from build123d import *

# Parameters (mm, degrees)
SKETCH_1_R               = 17.25
EXTRUDE_1_DEPTH          = 14
SKETCH_2_R               = 31
EXTRUDE_2_DEPTH          = 10
CUT_EXTRUDE_1_DEPTH      = 50.979995998
CUT_EXTRUDE_1_DEPTH_BACK = 50.979995998
SKETCH_3_W               = 21
SKETCH_3_H               = 21
EXTRUDE_3_DEPTH          = 20
SKETCH_5_W               = 21
SKETCH_5_H               = 21
CUT_EXTRUDE_2_DEPTH      = 20
SKETCH_6_R               = 1.65
CUT_EXTRUDE_3_DEPTH      = 56
EXTRUDE_4_DEPTH          = 5


with BuildPart() as part:
    # 草图1 → 凸台-拉伸1 (new body)
    with BuildSketch(Plane.XY):
        Circle(SKETCH_1_R)
    extrude(amount=EXTRUDE_1_DEPTH)

    # 草图2 → 凸台-拉伸2 (add)
    with BuildSketch(Plane.XY.offset(14)):
        Circle(SKETCH_2_R)
    extrude(amount=EXTRUDE_2_DEPTH)

    # 草图3 → 切除-拉伸1 (cut, two sides: drawn at the far end of the back side and taken through both)
    with BuildSketch(Plane(origin=(0, 0, 0), x_dir=(-1, 0, 0), z_dir=(0, 0, -1)).offset(-CUT_EXTRUDE_1_DEPTH_BACK)):
        Rectangle(SKETCH_3_W, SKETCH_3_H)
    extrude(amount=CUT_EXTRUDE_1_DEPTH + CUT_EXTRUDE_1_DEPTH_BACK, mode=Mode.SUBTRACT)

    # 草图4 → 凸台-拉伸3 (add)
    with BuildSketch(Plane.XY.offset(24)):
        with BuildLine():
            Line((-12.959637187, 15.233115373), (13.493683466, 14.762130826))
            ThreePointArc((13.493683466, 14.762130826), (20, 0), (13.493683466, -14.762130826))
            Line((13.493683466, -14.762130826), (-12.959637187, -15.233115373))
            ThreePointArc((-12.959637187, -15.233115373), (-20, 0), (-12.959637187, 15.233115373))
        make_face()
    extrude(amount=EXTRUDE_3_DEPTH)

    # 草图5 → 切除-拉伸2 (cut)
    with BuildSketch(Plane(origin=(0, 0, 24), x_dir=(-1, 0, 0), z_dir=(0, 0, -1))):
        Rectangle(SKETCH_5_W, SKETCH_5_H)
    extrude(amount=-CUT_EXTRUDE_2_DEPTH, mode=Mode.SUBTRACT)

    # 草图6 → 切除-拉伸3 (cut)
    with BuildSketch(Plane(origin=(0.267023139, 14.9976231, 0), x_dir=(0.9998415399853875, -0.017801542619919335, 0), z_dir=(0.017801542619919338, 0.9998415399853876, 0))):
        with Locations((0, -34)):
            Circle(SKETCH_6_R)
    extrude(amount=-CUT_EXTRUDE_3_DEPTH, mode=Mode.SUBTRACT)

    # 草图8 → 凸台-拉伸4 (add)
    with BuildSketch(Plane.XY.offset(44)):
        with BuildLine():
            Line((-12.959637187, -15.233115373), (13.493683466, -14.762130826))
            ThreePointArc((13.493683466, -14.762130826), (20, 0), (13.493683466, 14.762130826))
            Line((13.493683466, 14.762130826), (-12.959637187, 15.233115373))
            ThreePointArc((-12.959637187, 15.233115373), (-20, 0), (-12.959637187, -15.233115373))
        make_face()
    extrude(amount=EXTRUDE_4_DEPTH)


solid = part.part
CAD build for the part. Positions are in the model's coordinates, mm. A direction names the side the tool comes from. Give positions to 0.01 mm unless a question says otherwise; leave off trailing zeros. Loops run counter-clockwise (first coordinate to the right, second up) from the corner with the lowest first, then second, coordinate; pieces in that order, holes last. Notation, with made-up numbers: M 71,86 L 85,86 A18 cw 85,99 Z; hole C -2,13 d7. An arc over 180 degrees is marked long. Answer in a Markdown table with one row per item. Add a question column.
Item 1: Band-saw the part on C-C on z = 13. Give the cut face in (x, y), then the cut area to 3 significant figures.
Item 2: Band-saw the part on A-A on z = 39. Give the cut face in (x, y), then the cut area to 3 significant figures.
Item 3: Tool access for faces 5 (the face through (20, 0, 36)), 6 (the face through (-4.036, 30.736, 18.93)), 7 (the face through (10.5, 0, 22)): list every direction of +Z, -Z, +X, -X, +Y, -Y with a clear straight run to the whole face (end or side of a thin tool).
Item 4: Probe probe 1 along X at (y, z) = (-0.5, 9); probe 2 along X at (y, z) = (4, 2); probe 3 along Y at (x, z) = (0, 42.5). List the from-to ranges inside material, lowest first.
Item 5: Band-saw the part on B-B on y = 0. Give the cut face in (x, z).
Item 6: Mould opens along Y. For faces 1 (the face through (0, -20, 24)), 2 (the face through (0, -10.5, 22)), 3 (the face through (0, 10.5, 22)), 4 (the face through (-20, 0, 36)) say: +Y half, -Y half, draft (parallel to the pull), parting line (faces both ways), or undercut.
Item 7: Band-saw the part on D-D on x = 0. Give the number of separate pieces and of enclosed holes in the cut face, then the cut area to 3 significant figures.
Item 8: Drop flat-ended pins along their axis: P1, Ø1, axis at x = 6.5, z = 6, coming from the +Y side; P2, Ø4, axis at y = 11.5, z = 44, coming from the -X side; P3, Ø10, axis at x = 19.5, y = -12, coming from the -Z side. Give the stop position or say it passes through.
Reply:
| question | item | result |
|---|---|---|
| 1 | outline | C 0,0 d34.5; hole M -10.5,-10.5 L 10.5,-10.5 L 10.5,10.5 L -10.5,10.5 Z |
| 1 | area | 494 mm^2 |
| 2 | outline | M -12.96,-15.23 L 13.49,-14.76 A20 ccw 13.49,14.76 L -12.96,15.23 A20 ccw Z; hole M -10.5,-10.5 L 10.5,-10.5 L 10.5,10.5 L -10.5,10.5 Z |
| 2 | area | 634 mm^2 |
| 3 | face 5 | +Z, +X |
| 3 | face 6 | +Z, -Z |
| 3 | face 7 | -Z |
| 4 | probe 1 | x = -17.24 to -10.5, 10.5 to 17.24 |
| 4 | probe 2 | x = -16.78 to -10.5, 10.5 to 16.78 |
| 4 | probe 3 | y = -15 to -10.5, 10.5 to 15 |
| 5 | outline | M -31,14 L -17.25,14 L -17.25,0 L -10.5,0 L -10.5,44 L 10.5,44 L 10.5,0 L 17.25,0 L 17.25,14 L 31,14 L 31,24 L 20,24 L 20,49 L -20,49 L -20,24 L -31,24 Z |
| 6 | face 1 | draft |
| 6 | face 2 | undercut |
| 6 | face 3 | undercut |
| 6 | face 4 | parting line |
| 7 | separate pieces | 3 |
| 7 | enclosed holes | 0 |
| 7 | area | 900 mm^2 |
| 8 | P1 | stops at y = 16.17 |
| 8 | P2 | stops at x = -17.6 |
| 8 | P3 | stops at z = 14 |
